Autodesk Inventor part; units mm, degrees
ref_plane "YZ Plane" through (0, 0, 0) normal (1, 0, 0) x (0, 1, 0)
ref_plane "XZ Plane" through (0, 0, 0) normal (0, 1, 0) x (-1, 0, 0)
ref_plane "XY Plane" through (0, 0, 0) normal (0, 0, 1) x (1, 0, 0)
sketch "Sketch1" plane through (0, 0, 0) normal (0, 1, 0) x (-1, 0, 0)
  line L0 (0, 0) -> (-90, 0)
  line L1 (-90, 0) -> (-90, -200)
  line L2 (-90, -200) -> (0, -200)
  line L3 (0, -200) -> (0, 0)
  line L4 (2.5, -202.5) -> (-92.5, -202.5)
  line L5 (-92.5, -202.5) -> (-92.5, 2.5)
  line L6 (-92.5, 2.5) -> (2.5, 2.5)
  line L7 (2.5, 2.5) -> (2.5, -202.5)
  line L8 (2.5, -202.5) -> (-92.5, 2.5) construction
  line L9 (-92.5, -202.5) -> (2.5, 2.5) construction
  point P0 (-45, -100)
  dimension "d0" = 90
  dimension "d1" = 200
  dimension "d2" = 95
  dimension "d3" = 205
extrude "Extrusion1" add sketch "Sketch1" along normal blind 100
sketch "Sketch2" plane through (0, 0, 0) normal (0, -1, 0) x (1, 0, 0)
  line L0 (92.5, 2.5) -> (-2.5, 2.5)
  line L1 (-2.5, 2.5) -> (-2.5, -202.5)
  line L2 (-2.5, -202.5) -> (92.5, -202.5)
  line L3 (92.5, -202.5) -> (92.5, 2.5)
  point P0 (0, 0)
extrude "Extrusion2" add sketch "Sketch2" along normal blind 2.5
sketch "Sketch3" plane through (-2.5, 100, 2.5) normal (0, 0, 1) x (1, 0, 0)
  line L0 (2.5, -100) -> (17.5, -100)
  line L1 (92.5, -100) -> (2.5, -100)
  line L2 (17.5, -100) -> (17.5, -90)
  line L3 (17.5, -90) -> (77.5, -90)
  line L4 (77.5, -90) -> (77.5, -78)
  line L5 (77.5, -78) -> (17.5, -90)
  line L6 (17.5, -90) -> (17.5, -80)
  line L7 (17.5, -80) -> (17.5, -70)
  line L8 (17.5, -70) -> (23, -70)
  circle A0 centre (23, -70) radius 5.5
  line L9 (28.5, -70) -> (28.5, -76.5)
  line L10 (96.033, -55.3934) -> (23, -70)
  line L11 (17.6068, -71.0786) -> (17.5, -71.1)
  line L12 (23, -70) -> (38, -70)
  line L13 (38, -70) -> (38, -67)
  circle A1 centre (38, -67) radius 5.5
  line L14 (38, -67) -> (53, -67)
  line L15 (53, -67) -> (53, -64)
  line L16 (53, -64) -> (68, -64)
  line L17 (68, -64) -> (68, -61)
  circle A2 centre (53, -64) radius 5.5
  circle A3 centre (68, -61) radius 5.5
  line L18 (32.6068, -68.0786) -> (32.6068, -76.5)
  line L19 (43.5, -67) -> (43.5, -73.5)
  line L20 (47.6068, -65.0786) -> (47.6068, -73.5)
  line L21 (58.5, -64) -> (58.5, -70.5)
  line L22 (62.6068, -62.0786) -> (62.6068, -70.5)
  line L23 (73.3932, -59.9214) -> (73.3932, -78.8214)
  line L24 (28.5, -76.5) -> (32.6068, -76.5)
  line L25 (43.5, -73.5) -> (47.6068, -73.5)
  line L26 (58.5, -70.5) -> (62.6068, -70.5)
  circle A4 centre (30.5534, -74.4466) radius 2.0534
  circle A5 centre (45.5534, -71.4466) radius 2.0534
  circle A6 centre (60.5534, -68.4466) radius 2.0534
  point P0 (32.6068, -74.4466)
  point P1 (28.5, -74.4466)
  point P2 (62.6068, -68.4466)
  point P3 (58.5, -68.4466)
  point P4 (47.6068, -71.4466)
  point P5 (43.5, -71.4466)
  dimension "d9" = 15
  dimension "d10" = 10
  dimension "d11" = 90
  dimension "d12" = 60
  dimension "d13" = 12
  dimension "d14" = 10
  dimension "d15" = 10
  dimension "d16" = 5.5
  dimension "d17" = 6.5
  dimension "d18" = 15
  dimension "d19" = 11
  dimension "d20" = 15
  dimension "d21" = 15
  dimension "d22" = 11
  dimension "d23" = 11
  dimension "d24" = 6.5
  dimension "d25" = 6.5
extrude "Extrusion3" cut sketch "Sketch3" against normal blind 15 contours L6 L7 L11 A0 L9 L24 L18 L12 A1 L19 L25 L20 L14 A2 L21 L26 L22 L16 A3 L23 L5 | A3 L16 L17 L10 L23 | A3 L10 L17 L16 | L16 L22 A3 | L10 A3 | A0 L10 L8 | L8 L12 A0 | L10 A0 L12 | A2 L14 L15 L16 | L16 L10 A2 | L22 L26 A6 | L10 A2 | A1 L10 | L10 L13 L12 A1 | A1 L12 L18 | A4 L24 L9 | L15 L14 A2 L10 | L14 L20 A2 | A6 L26 L21 | L14 A1 L12 L13 | L10 A1 L14 | L18 L24 A4 | L20 L25 A5 | A5 L25 L19
sketch "Sketch4" plane through (-2.5, 100, -202.5) normal (-1, 0, 0) x (0, 0, 1)
  line L0 (202.5, -100) -> (2.5, -100)
  line L1 (2.5, -100) -> (2.5, -90)
  line L2 (2.5, -100) -> (2.5, 0)
  line L3 (2.5, -90) -> (54.5, -90)
  line L4 (54.5, -90) -> (54.5, -48)
  circle A0 centre (54.5, -48) radius 5
  line L5 (54.5, -48) -> (149.5, -48)
  circle A1 centre (149.5, -48) radius 5
  dimension "d28" = 10
  dimension "d29" = 52
  dimension "d30" = 42
  dimension "d31" = 10
  dimension "d32" = 95
  dimension "d33" = 10
extrude "Extrusion4" cut sketch "Sketch4" against normal through all
equation "\"d26\" = d20"
properties part number "Box"
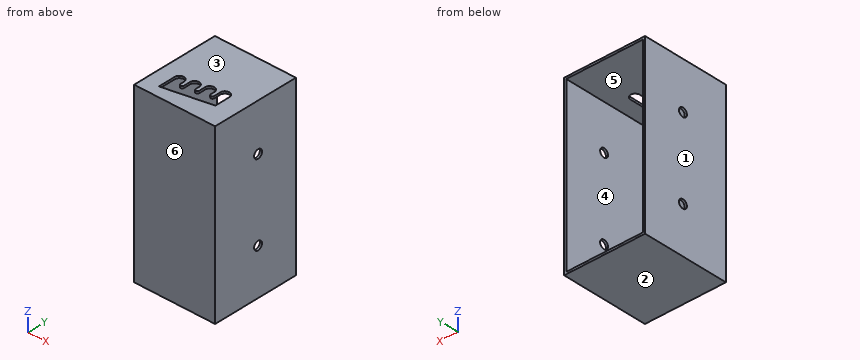
Geometry: final body of the model. Coordinates: model frame, mm. Face numbers are marked on the shaded views. A direction names the side the tool comes from. Give positions to 0.01 mm unless a question says otherwise; leave off trailing zeros. Loops run counter-clockwise (first coordinate to the right, second up) from the corner with the lowest first, then second, coordinate; pieces in that order, holes last. Notation, with made-up numbers: (-30.5, 72.25) -> (20.5, 72.25) arc R27 ccw to (20.5, 91.25) -> close; hole circle Ø4 at (75.5, -2). An arc over 180 degrees is marked (long way). Use one line per item in the form item = value.
Item 1: Section query D-D on z = -13.5. Output: boundary loops of the cut face in (x, y), and give its area (4 significant figures).
A:
outline = (-2.5, -2.5) -> (92.5, -2.5) -> (92.5, 100) -> (90, 100) -> (90, 0) -> (0, 0) -> (0, 100) -> (-2.5, 100) -> close
area = 737.5 mm^2
Item 2: Pin query (flat end, axial travel): P1, Ø5, axis at x = 67, z = -89.5, coming from the +Y side; P2, Ø10, axis at x = 20.5, y = 30, coming from the +Z side; P3, Ø9, axis at y = 52, z = -53, coming from the +X side. Return the tip coordinate at first contact, or that it passes through.
A:
P1 = 0
P2 = -200
P3 = through
Item 3: Access query for the marked faces 5 and 6. Directions: +Z, -Z, +X, -X, +Y, -Y. A direction counts if a zero-diameter tool reaches every point of the face in a straight line with its end or side. Return the directions, or none.
A:
face_5 = +Y
face_6 = +Z, -Z, +X, -X, -Y
Item 4: Line query: probe 1 along X at (y, z) = (44, -47.5); probe 2 along X at (y, z) = (30, 1.55); probe 3 along Z at (x, y) = (-1, 52). Output: solid intervals per line, ascending.
A:
probe_1 = -2.5 to 0, 90 to 92.5
probe_2 = -2.5 to 15, 26 to 30.11, 41 to 45.11, 56.71 to 59.4, 70.89 to 92.5
probe_3 = -202.5 to -153, -143 to -58, -48 to 2.5
Item 5: Section query A-A on x = 65.5. Output: boundary loops of the cut face in (y, z), and give its area (4 significant figures).
A:
outline = (-2.5, -202.5) -> (100, -202.5) -> (100, -200) -> (0, -200) -> (0, 0) -> (20.1, 0) -> (20.1, 2.5) -> (-2.5, 2.5) -> close; (44.5, 0) -> (100, 0) -> (100, 2.5) -> (44.5, 2.5) -> close
area = 951.5 mm^2
Item 6: Section query C-C on y = 78.5. Output: boundary loops of the cut face in (x, z).
A:
outline = (-2.5, -202.5) -> (92.5, -202.5) -> (92.5, 2.5) -> (-2.5, 2.5) -> close; hole (0, -200) -> (90, -200) -> (90, 0) -> (0, 0) -> close
Item 7: Section query B-B on z = -148. Output: boundary loops of the cut face in (x, y).
A:
outline = (-2.5, -2.5) -> (92.5, -2.5) -> (92.5, 47) -> (90, 47) -> (90, 0) -> (0, 0) -> (0, 47) -> (-2.5, 47) -> close; (-2.5, 57) -> (0, 57) -> (0, 100) -> (-2.5, 100) -> close; (90, 57) -> (92.5, 57) -> (92.5, 100) -> (90, 100) -> close
Item 8: Draft query along Z for the marked faces 1, 2, 3 and 4. Return one class per face: pulls with the +Z half, pulls with the -Z half, needs draft (parallel to the pull), parting line crosses it, or undercut.
A:
face_1 = needs draft
face_2 = pulls with the -Z half
face_3 = pulls with the +Z half
face_4 = undercut
